```python
from build123d import *

# Parameters (mm, degrees)
CROQUIS1_W              = 145
CROQUIS1_H              = 131.5
SALIENTE_EXTRUIR1_DEPTH = 40
VACIADO1_T              = -1
CROQUIS2_W              = 143
CROQUIS2_H              = 78
CORTAR_EXTRUIR1_DEPTH   = 160
CROQUIS3_W              = 78
CROQUIS3_H              = 129.5
CORTAR_EXTRUIR2_DEPTH   = 180


with BuildPart() as part:
    # Croquis1 → Saliente-Extruir1 (new, symmetric)
    with BuildSketch(Plane.XY):
        Rectangle(CROQUIS1_W, CROQUIS1_H)
    extrude(amount=SALIENTE_EXTRUIR1_DEPTH, both=True)

    # Vaciado1
    vaciado1_openings = [part.faces().sort_by_distance(p)[0] for p in [
        (0, 0, 40),
    ]]
    offset(amount=VACIADO1_T, openings=vaciado1_openings, kind=Kind.INTERSECTION)

    # Croquis2 → Cortar-Extruir1 (cut)
    with BuildSketch(Plane(origin=(0, 65.75, 0), x_dir=(1, 0, 0), z_dir=(0, 1, 0))):
        Rectangle(CROQUIS2_W, CROQUIS2_H)
    extrude(amount=-CORTAR_EXTRUIR1_DEPTH, mode=Mode.SUBTRACT)

    # Croquis3 → Cortar-Extruir2 (cut)
    with BuildSketch(Plane(origin=(72.5, 0, 0), x_dir=(0, 0, -1), z_dir=(1, 0, 0))):
        Rectangle(CROQUIS3_W, CROQUIS3_H)
    extrude(amount=-CORTAR_EXTRUIR2_DEPTH, mode=Mode.SUBTRACT)


solid = part.part
```
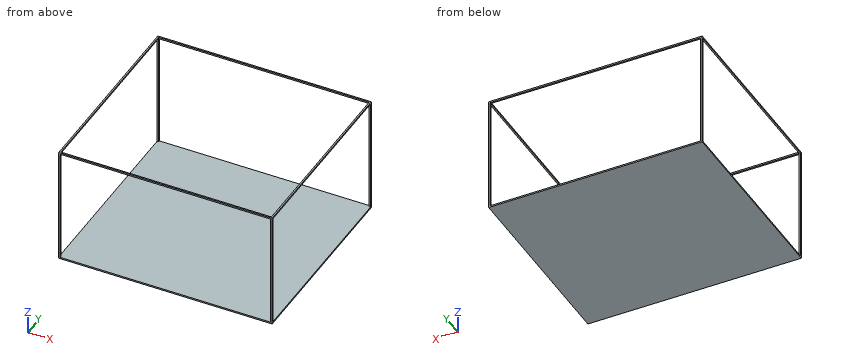
Input: part model. Units: mm. Frame: model coordinates. Round coordinates to 2 decimals unless told otherwise and drop trailing zeros. Loops run counter-clockwise (first coordinate to the right, second up) from the corner with the lowest first, then second, coordinate; pieces in that order, holes last. Notation, with made-up numbers: (12, 17) - (71, 17) arc R28 cw to (71, 51) - close; hole circle Ø8 at (15.5, 61). An arc over 180 degrees is marked (long way). One line per item, written item: value. Start each with the question number.
(1) Ray query, line 1 (Z direction, x = 16.5, y = 37). Return the intervals inside material, ascending. Write a range as [from, to].
(2) Section B-B, the plane z = 26. Return loops of the section in (x, y).
(3) Section C-C, the plane y = -29. Return loops of the section in (x, z), plus the area to 3 significant figures.
(4) Section A-A, the plane x = -55.5. Return loops of the section in (y, z), plus the area to 4 significant figures.
(5) Contact query for a flat-ended pin moving along its axis: P1, Ø4, axis at x = -5, y = 32, coming from the +Z side. Output: stop coordinate, or through.
Results below:
1. line 1: [-40, -39]
2. outline: (-72.5, -65.75) - (-71.5, -65.75) - (-71.5, -64.75) - (-72.5, -64.75) - close; (-72.5, 64.75) - (-71.5, 64.75) - (-71.5, 65.75) - (-72.5, 65.75) - close; (71.5, -65.75) - (72.5, -65.75) - (72.5, -64.75) - (71.5, -64.75) - close; (71.5, 64.75) - (72.5, 64.75) - (72.5, 65.75) - (71.5, 65.75) - close
3. outline: (-72.5, -40) - (72.5, -40) - (72.5, -39) - (-72.5, -39) - close; (-72.5, 39) - (-71.5, 39) - (-71.5, 40) - (-72.5, 40) - close; (71.5, 39) - (72.5, 39) - (72.5, 40) - (71.5, 40) - close
3. area: 147 mm^2
4. outline: (-65.75, -40) - (65.75, -40) - (65.75, -39) - (-65.75, -39) - close; (-65.75, 39) - (-64.75, 39) - (-64.75, 40) - (-65.75, 40) - close; (64.75, 39) - (65.75, 39) - (65.75, 40) - (64.75, 40) - close
4. area: 133.5 mm^2
5. P1: z = -39
